Drawing for the job (mm, zero at the part's lowest x, y, z). A direction names the side the tool comes from. Round coordinates to 2 decimals unless told otherwise and drop trailing zeros. Write each loop counter-clockwise with the first axis right and the second up, starting at its lowest first coordinate (ties: lowest second). Pieces come first, ordered by that corner, then holes. Notation, with made-up numbers: M 64,77.5 L 120,77.5 A32 cw 120,115.5 Z; hole C 50,36 d11. An arc over 180 degrees is marked long. Use a Markdown table: item, result.
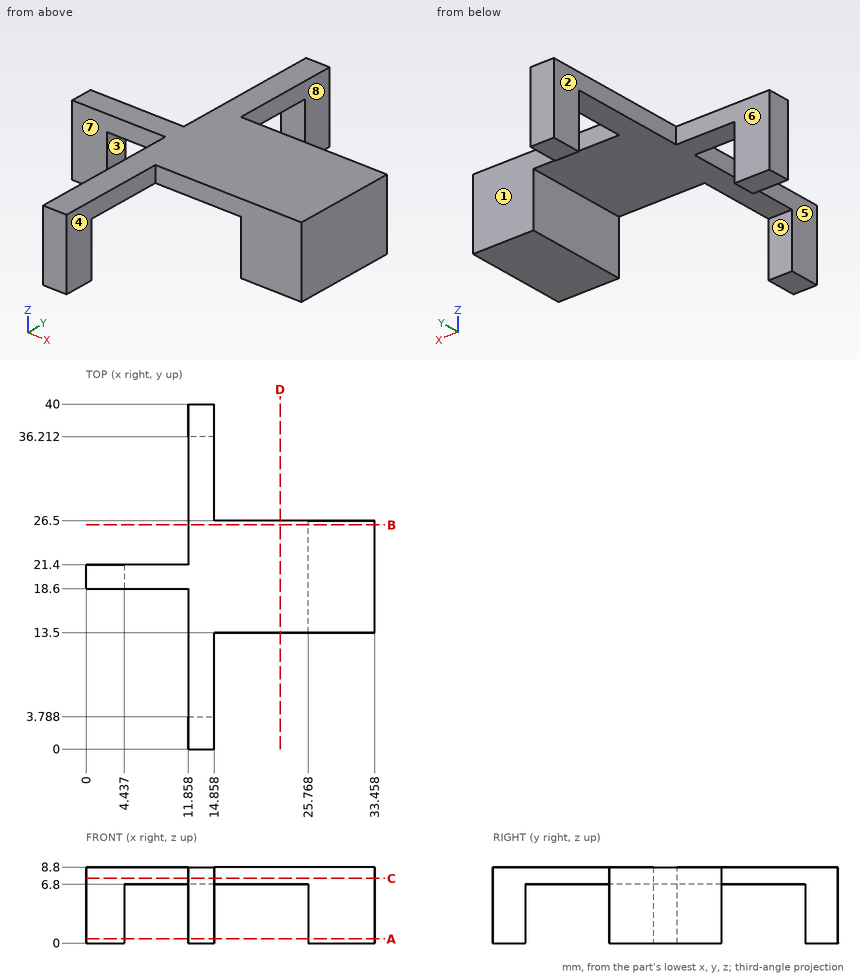
Q1. Cut at A-A on z = 0.5. Give the cut face in (x, y).
Response values:
| item | result |
|---|---|
| outline | M 0,18.6 L 4.44,18.6 L 4.44,21.4 L 0,21.4 Z; M 11.86,0 L 14.86,0 L 14.86,3.79 L 11.86,3.79 Z; M 11.86,36.21 L 14.86,36.21 L 14.86,40 L 11.86,40 Z; M 25.77,13.5 L 33.46,13.5 L 33.46,26.5 L 25.77,26.5 Z |
Q2. Cut at D-D on x = 22.5. Give the cut face in (y, z).
Response values:
| item | result |
|---|---|
| outline | M 13.5,6.8 L 26.5,6.8 L 26.5,8.8 L 13.5,8.8 Z |
Q3. Drill centre lines: L1, parallel to Y at x = 14, z = 2.75; L2, parallel to X at y = 21.5, z = 1.25; L3, parallel to X at y = 31, z = 7.5. Where is each one in solid material? Low to high.
Response values:
| item | result |
|---|---|
| L1 | y = 0 to 3.79, 36.21 to 40 |
| L2 | x = 25.77 to 33.46 |
| L3 | x = 11.86 to 14.86 |
Q4. Which spindle directions (+Z, -Z, +X, -X, +Y, -Y) get a long thin tool onto all of the face, cutting with end or side? Do the marked faces 1, 2, 3, 4 and 5. Say none if no direction does.
Response values:
| item | result |
|---|---|
| face 1 | +Z, -Z, +X, +Y |
| face 2 | +Z, -Z, -X, +Y |
| face 3 | -Z, +Y, -Y |
| face 4 | +Z, -Z, +X, -Y |
| face 5 | +Z, -Z, -X, -Y |
Q5. Two-plate mould, pull along Y, no slides. Class the marked faces 6, 7, 8 and 9: +Y half, -Y half, draft (parallel to the pull), parting line (faces both ways), or undercut.
Response values:
| item | result |
|---|---|
| face 6 | +Y half |
| face 7 | -Y half |
| face 8 | draft |
| face 9 | undercut |
Q6. Cut at C-C on z = 7.5. Give the cut face in (x, y).
Response values:
| item | result |
|---|---|
| outline | M 0,18.6 L 11.86,18.6 L 11.86,0 L 14.86,0 L 14.86,13.5 L 33.46,13.5 L 33.46,26.5 L 14.86,26.5 L 14.86,40 L 11.86,40 L 11.86,21.4 L 0,21.4 Z |
Q7. Cut at B-B on y = 26. Give the cut face in (x, z).
Response values:
| item | result |
|---|---|
| outline | M 11.86,6.8 L 25.77,6.8 L 25.77,0 L 33.46,0 L 33.46,8.8 L 11.86,8.8 Z |
Q8. Drop flat-ended pins along their axis: P1, Ø1.5, axis at y = 16, z = 6, coming from the -X side; P2, Ø4.5, axis at y = 34.5, z = 3.5, coming from the +X side; P3, Ø10, axis at x = 11, y = 28, coming from the -Z side. Give the stop position or say it passes through.
Response values:
| item | result |
|---|---|
| P1 | stops at x = 25.77 |
| P2 | stops at x = 14.86 |
| P3 | stops at z = 6.8 |
